```python
from build123d import *

# Parameters (mm, degrees)
F0_W     = 4
F0_H     = 2.9
F0_W_2   = 3
F0_H_2   = 1.9
F0_R     = 1.5
F0_R_2   = 5.5
F1_DEPTH = 2
F2_DEPTH = 2


with BuildPart() as f1:
    # F0 (on Right) → F1 (new body)
    with BuildSketch(Plane.YZ):
        with Locations((-13, -9.45)):
            Rectangle(F0_W, F0_H)
        with Locations((13, -9.45)):
            Rectangle(F0_W, F0_H)
        with Locations((-7.80476, 38.95)):
            Rectangle(F0_W_2, F0_H_2)
        with Locations((7.80476, 38.95)):
            Rectangle(F0_W_2, F0_H_2)
        Polygon((-9.30476, 38), (-9.30476, 35), (9.30476, 35), (9.30476, 38), (6.30476, 38), (-6.30476, 38), align=None)
        Polygon((-15, -6), (-15, -8), (-11, -8), (11, -8), (15, -8), (15, -6), (13, -6), (13, -3), (15, -3), (15, 3), (13, 3), (13, 6), (15, 6), (15, 8), (-15, 8), (-15, 6), (-13, 6), (-13, 3), (-15, 3), (-15, -3), (-13, -3), (-13, -6), align=None)
        with Locations((-9, 0)):
            Circle(F0_R, mode=Mode.SUBTRACT)
        Circle(F0_R_2, mode=Mode.SUBTRACT)
        with Locations((9, 0)):
            Circle(F0_R, mode=Mode.SUBTRACT)
        Polygon((-9.30476, 35), (-15, 8), (15, 8), (9.30476, 35), align=None)
        with BuildLine():
            ThreePointArc((3.6272711829, 30), (4.8871178359, 29.5533146529), (5.5842094494, 28.4127864109))
            Line((5.5842094494, 28.4127864109), (8.326362042, 15.4127864109))
            ThreePointArc((8.326362042, 15.4127864109), (7.9227384284, 13.740153347), (6.3694237755, 13))
            Line((6.3694237755, 13), (-6.3694237755, 13))
            ThreePointArc((-6.3694237755, 13), (-7.9227384284, 13.740153347), (-8.326362042, 15.4127864109))
            Line((-8.326362042, 15.4127864109), (-5.5842094494, 28.4127864109))
            ThreePointArc((-5.5842094494, 28.4127864109), (-4.8871178359, 29.5533146529), (-3.6272711829, 30))
            Line((-3.6272711829, 30), (3.6272711829, 30))
        make_face(mode=Mode.SUBTRACT)
    extrude(amount=F1_DEPTH)

    # F0 (on Right) → F2 (join)
    with BuildSketch(Plane.YZ):
        Polygon((-9.30476, 35), (-15, 8), (15, 8), (9.30476, 35), align=None)
        with BuildLine():
            ThreePointArc((3.6272711829, 30), (4.8871178359, 29.5533146529), (5.5842094494, 28.4127864109))
            Line((5.5842094494, 28.4127864109), (8.326362042, 15.4127864109))
            ThreePointArc((8.326362042, 15.4127864109), (7.9227384284, 13.740153347), (6.3694237755, 13))
            Line((6.3694237755, 13), (-6.3694237755, 13))
            ThreePointArc((-6.3694237755, 13), (-7.9227384284, 13.740153347), (-8.326362042, 15.4127864109))
            Line((-8.326362042, 15.4127864109), (-5.5842094494, 28.4127864109))
            ThreePointArc((-5.5842094494, 28.4127864109), (-4.8871178359, 29.5533146529), (-3.6272711829, 30))
            Line((-3.6272711829, 30), (3.6272711829, 30))
        make_face(mode=Mode.SUBTRACT)
        Polygon((-15, -6), (-15, -8), (-11, -8), (11, -8), (15, -8), (15, -6), (13, -6), (13, -3), (15, -3), (15, 3), (13, 3), (13, 6), (15, 6), (15, 8), (-15, 8), (-15, 6), (-13, 6), (-13, 3), (-15, 3), (-15, -3), (-13, -3), (-13, -6), align=None)
        with Locations((-9, 0)):
            Circle(F0_R, mode=Mode.SUBTRACT)
        Circle(F0_R_2, mode=Mode.SUBTRACT)
        with Locations((9, 0)):
            Circle(F0_R, mode=Mode.SUBTRACT)
        with Locations((-13, -9.45)):
            Rectangle(F0_W, F0_H)
        with Locations((13, -9.45)):
            Rectangle(F0_W, F0_H)
        with Locations((7.80476, 38.95)):
            Rectangle(F0_W_2, F0_H_2)
        Polygon((-9.30476, 38), (-9.30476, 35), (9.30476, 35), (9.30476, 38), (6.30476, 38), (-6.30476, 38), align=None)
        with Locations((-7.80476, 38.95)):
            Rectangle(F0_W_2, F0_H_2)
    extrude(amount=F2_DEPTH)


solid = f1.part
```
Source: CAD feature listing. Evaluate the final solid. Frame: model axes, mm. A direction names the side the tool comes from. Round coordinates to 2 decimals unless told otherwise and drop trailing zeros. Write each loop counter-clockwise with the first axis right and the second up, starting at its lowest first coordinate (ties: lowest second). Pieces come first, ordered by that corner, then holes. Notation, with made-up numbers: M 42,-23.75 L 58,-23.75 A12 cw 58,-14.75 Z; hole C 67,61.25 d3. An arc over 180 degrees is marked long. Use CSV: the item, a comma, the result in double quotes. Start each with the question number.
Q1. Pull-direction query (Y, two-part tool) for faces 6 (the face through (1, 15, -8)), 7 (the face through (0.99, -10.5, 0.07)), 8 (the face through (1, -14, -6)), 9 (the face through (1, -15, -8)); classes: +Y half, -Y half, draft (parallel to the pull), parting line (faces both ways), or undercut.
Q2. Access query for faces 1 (the face through (1, 14, 3)), 2 (the face through (1, -14, 3)), 3 (the face through (1, -6.305, 39)), 4 (the face through (1, -11, -9)), 5 (the face through (0.986, -7.907, 13.721)). Directions: +Z, -Z, +X, -X, +Y, -Y. A direction counts if a zero-diameter tool reaches every point of the face in a straight line with its end or side. Return the directions, or none.
Q3. Cut plane C-C on z = 16. Output: boundary loops of the cut face in (x, y).
Q4. Cut plane D-D on x = 0.95. Count the separate pieces of the cut face and the enclosed holes in it, plus the area to 3 significant figures.
Q5. Line query: line 1 (Z direction, x = 1.1, y = 5); line 2 (Z direction, x = 1, y = -9); line 3 (Z direction, x = 0.35, y = 4.5). Output: solid intervals per line, ascending. Write a range as from..to.
Q6. First-contact query: P1, Ø0.6, axis at x = 0.5, y = -5, coming from the -Z side; P2, Ø1.8, axis at y = -9, z = 0, coming from the -X side; P3, Ø0.6, axis at x = 0.5, z = 4.5, coming from the -Y side. Flat tips, straight axial feed; report the tip coordinate or a pass-through.
Q7. Cut plane A-A on z = 0. Output: boundary loops of the cut face in (x, y).
Q8. Cut plane B-B on y = 0. Output: boundary loops of the cut face in (x, z), plus the area to 3 significant figures.
Results found:
1,face 6,"+Y half"
1,face 7,"undercut"
1,face 8,"draft"
1,face 9,"-Y half"
2,face 1,"+X, -X, +Y"
2,face 2,"+X, -X, -Y"
2,face 3,"+Z, +X, -X"
2,face 4,"-Z, +X, -X"
2,face 5,"+X, -X"
3,outline,"M 0,-13.31 L 2,-13.31 L 2,-8.2 L 0,-8.2 Z; M 0,8.2 L 2,8.2 L 2,13.31 L 0,13.31 Z"
4,separate pieces,"1"
4,enclosed holes,"4"
4,area,"858 mm^2"
5,line 1,"-8..-2.29, 2.29..13, 29.45..38"
5,line 2,"-8..-1.5, 1.5..39.9"
5,line 3,"-8..-3.16, 3.16..13, 29.8..38"
6,P1,"z = -8"
6,P2,"through"
6,P3,"y = -13"
7,outline,"M 0,-15 L 2,-15 L 2,-10.5 L 0,-10.5 Z; M 0,-7.5 L 2,-7.5 L 2,-5.5 L 0,-5.5 Z; M 0,5.5 L 2,5.5 L 2,7.5 L 0,7.5 Z; M 0,10.5 L 2,10.5 L 2,15 L 0,15 Z"
8,outline,"M 0,-8 L 2,-8 L 2,-5.5 L 0,-5.5 Z; M 0,5.5 L 2,5.5 L 2,13 L 0,13 Z; M 0,30 L 2,30 L 2,38 L 0,38 Z"
8,area,"36.0 mm^2"
